The listing builds one solid part. Answer for the finished solid, in the listing's coordinates (mm). Round coordinates to 2 decimals unless told otherwise and drop trailing zeros. Order: outer loops, then holes, each group sorted by start corner. A loop starts at its lowest first (then second) coordinate and runs counter-clockwise, first axis right, second up. Notation, with made-up numbers: (54, -20) - (70, -20) arc R27 cw to (70, 0) - close; hole circle Ø6 at (50.25, 86.5). An arc over 180 degrees is marked (long way). Use CSV: the item, a comma, the result in double quotes. Start each with the question number.
Item 1: Straight lines are drawn through the part: line 1 along X through (y, z) = (22.5, -24); line 2 along X through (y, z) = (-4.5, -41); line 3 along Z through (x, y) = (-118, 36.5). For each, find the intervals that lie inside material, in ascending order. Write a range as [from, to].
Item 2: Find section A-A, the plane x = -44.5. Give the vertices of the cut face in (y, z), plus the area to 3 significant figures.
Item 3: Flat-ended cylindrical pins translate along their axes: P1, Ø5, axis at x = -74, z = -33, coming from the +Y side; P2, Ø5, axis at x = -126, y = -33.5, coming from the -Z side; P3, Ø5, axis at x = -59, y = -36, coming from the +Z side. Find the tip coordinate at first contact, or state that the pin passes through.
```python
from build123d import *

# Parameters (mm, degrees)
F0_R      = 50.811905
F1_DEPTH  = 82.55
F2_SIZE   = 50.8
F1_FACE_R = 50.811905
F3_DEPTH  = 152.4


with BuildPart() as f1:
    # F0 (on Right) → F1 (new body)
    with BuildSketch(Plane.YZ):
        Circle(F0_R)
    extrude(amount=F1_DEPTH)

    # F2
    f2_edges = [f1.edges().sort_by_distance(p)[0] for p in [
        (82.55, -50.811905, 0),
    ]]
    chamfer(f2_edges, length=F2_SIZE)

    # F1_face (on face) → F3 (join)
    with BuildSketch(Plane(origin=(0, 0, 0), x_dir=(0, 1, 0), z_dir=(-1, 0, 0))):
        Circle(F1_FACE_R)
    extrude(amount=F3_DEPTH)


solid = f1.part
```
Worked out:
1,line 1,"x = [-152.4, 49.66]"
1,line 2,"x = [-152.4, 41.32]"
1,line 3,"z = [-35.35, 35.35]"
2,outline,"circle Ø101.62 at (0, 0)"
2,area,"8,110 mm²"
3,P1,"stops at y = 40.64"
3,P2,"stops at z = -40.26"
3,P3,"stops at z = 38.2"
